Read the model definition and answer for the solid it produces. Units are mm, in the model's axes. Give positions to 0.01 mm unless a question says otherwise; leave off trailing zeros. Loops run counter-clockwise (first coordinate to the right, second up) from the corner with the lowest first, then second, coordinate; pieces in that order, holes last. Notation, with made-up numbers: (53.5, 30) - (88.5, 30) arc R19 ccw to (88.5, 34) - close; hole circle Ø4 at (55, -2). An arc over 180 degrees is marked (long way). Write item = value, one per line.
```python
from build123d import *

# Parameters (mm, degrees)
F0_W          = 158.75
F0_H          = 508
F1_DEPTH      = 158.75
F3_W          = 38.1
F3_H          = 114.3
F4_DEPTH      = 25.4
F2_W          = 31.75
F2_H          = 114.3
F5_DEPTH      = 25.4
F6_R          = 78.74
F7_SIZE       = 50.8
F8_W          = 38.1
F8_H          = 114.3
F9_DEPTH      = 25.4
F10_T2_ANGLE  = 90
F10_T4_ANGLE  = 90
F10_T6_ANGLE  = 90
F10_T8_ANGLE  = 90
F10_T12_DEPTH = 655.32
F10_T17_DEPTH = 655.32
F10_T23_DEPTH = 655.32
F10_T28_DEPTH = 655.32
F10_T33_DEPTH = 655.32
F10_T38_DEPTH = 655.32
F10_T43_DEPTH = 655.32
F10_T48_DEPTH = 655.32
F10_T53_DEPTH = 655.32
F10_T58_DEPTH = 655.32
F10_T63_DEPTH = 655.32
F10_T69_DEPTH = 655.32


# Not quite as in the source:
# - a fillet or chamfer that OpenCascade refuses, or shapes differently, is made with other operations: its cross-section is extruded or revolved along the edge and cut away or added


with BuildPart() as f1:
    # F0 (on Front) → F1 (new body)
    with BuildSketch(Plane.XZ):
        Rectangle(F0_W, F0_H)
    extrude(amount=F1_DEPTH)

    # F3 (on face) → F4 (join)
    with BuildSketch(Plane.YZ.offset(79.375)):
        with Locations((-79.375, 0)):
            Rectangle(F3_W, F3_H)
    extrude(amount=F4_DEPTH)

    # F2 (on face) → F5 (join)
    with BuildSketch(Plane.XZ.offset(158.75)):
        Rectangle(F2_W, F2_H)
    extrude(amount=F5_DEPTH)

    # F6
    f6_edges = [f1.edges().sort_by_distance(p)[0] for p in [
        (79.375, -79.375, 254),
        (-79.375, -79.375, 254),
        (0, 0, 254),
        (0, -158.75, 254),
    ]]
    fillet(f6_edges, radius=F6_R)

    # F7
    f7_edges = [f1.edges().sort_by_distance(p)[0] for p in [
        (-79.375, -79.375, -254),
        (79.375, -79.375, -254),
        (0, 0, -254),
        (0, -158.75, -254),
    ]]
    chamfer(f7_edges, length=F7_SIZE)

    # F8 (on face) → F9 (join)
    with BuildSketch(Plane(origin=(0, 0, 0), x_dir=(-1, 0, 0), z_dir=(0, 1, 0))):
        Rectangle(F8_W, F8_H)
    extrude(amount=F9_DEPTH)

    # F10: fillet of radius 79.248 on 4 edges, made by hand

    # F10_s1 → F10_t2 (revolve, cut)
    with BuildSketch(Plane.YZ.offset(0.127)):
        with BuildLine():
            ThreePointArc((-80.01, 254), (-135.6875879506, 230.9375879506), (-158.75, 175.26))
            Line((-158.75, 175.26), (-158.75, 254))
            Line((-158.75, 254), (-80.01, 254))
        make_face()
    revolve(axis=Axis((0.127, -79.502, 254), (0, 0, 1)), revolution_arc=F10_T2_ANGLE, mode=Mode.SUBTRACT)

    # F10_s3 → F10_t4 (revolve, cut)
    with BuildSketch(Plane.YZ.offset(-0.127)):
        with BuildLine():
            ThreePointArc((-78.74, 254), (-23.0624120494, 230.9375879506), (0, 175.26))
            Line((0, 175.26), (0, 254))
            Line((0, 254), (-78.74, 254))
        make_face()
    revolve(axis=Axis((-0.127, -79.248, 254), (0, 0, 1)), revolution_arc=F10_T4_ANGLE, mode=Mode.SUBTRACT)

    # F10_s5 → F10_t6 (revolve, cut)
    with BuildSketch(Plane.XZ.offset(79.502)):
        with BuildLine():
            ThreePointArc((-0.635, 254), (-56.3125879506, 230.9375879506), (-79.375, 175.26))
            Line((-79.375, 175.26), (-79.375, 254))
            Line((-79.375, 254), (-0.635, 254))
        make_face()
    revolve(axis=Axis((-0.127, -79.502, 254), (0, 0, 1)), revolution_arc=F10_T6_ANGLE, mode=Mode.SUBTRACT)

    # F10_s7 → F10_t8 (revolve, cut)
    with BuildSketch(Plane.XZ.offset(79.248)):
        with BuildLine():
            ThreePointArc((0.635, 254), (56.3125879506, 230.9375879506), (79.375, 175.26))
            Line((79.375, 175.26), (79.375, 254))
            Line((79.375, 254), (0.635, 254))
        make_face()
    revolve(axis=Axis((0.127, -79.248, 254), (0, 0, 1)), revolution_arc=F10_T8_ANGLE, mode=Mode.SUBTRACT)


with BuildPart() as f10_tool10:
    # F10_s11 → F10_t12 (new body)
    with BuildSketch(Plane.XY.offset(-401.32)):
        with BuildLine():
            ThreePointArc((0.127, 0), (56.1637981955, -23.2112018045), (79.375, -79.248))
            Line((79.375, -79.248), (79.375, 0))
            Line((79.375, 0), (0.127, 0))
        make_face()
    extrude(amount=F10_T12_DEPTH)

    split(bisect_by=Plane.XY.offset(-57.15), keep=Keep.BOTTOM)


with BuildPart() as f1_1:
    add(f1.part)

    # F10_t9: cut F10_tool10
    add(f10_tool10.part, mode=Mode.SUBTRACT)


with BuildPart() as f10_tool15:
    # F10_s16 → F10_t17 (new body)
    with BuildSketch(Plane.XY.offset(-401.32)):
        with BuildLine():
            ThreePointArc((0.127, 0), (56.1637981955, -23.2112018045), (79.375, -79.248))
            Line((79.375, -79.248), (79.375, 0))
            Line((79.375, 0), (0.127, 0))
        make_face()
    extrude(amount=F10_T17_DEPTH)

    split(bisect_by=Plane.YZ.offset(19.05), keep=Keep.TOP)

    split(bisect_by=Plane.XZ.offset(60.325), keep=Keep.BOTTOM)


with BuildPart() as f1_2:
    add(f1_1.part)

    # F10_t14: cut F10_tool15
    add(f10_tool15.part, mode=Mode.SUBTRACT)


with BuildPart() as f10_tool21:
    # F10_s22 → F10_t23 (new body)
    with BuildSketch(Plane.XY.offset(-401.32)):
        with BuildLine():
            ThreePointArc((0.127, 0), (56.1637981955, -23.2112018045), (79.375, -79.248))
            Line((79.375, -79.248), (79.375, 0))
            Line((79.375, 0), (0.127, 0))
        make_face()
    extrude(amount=F10_T23_DEPTH)

    split(bisect_by=Plane.XY.offset(57.15), keep=Keep.TOP)


with BuildPart() as f1_3:
    add(f1_2.part)

    # F10_t20: cut F10_tool21
    add(f10_tool21.part, mode=Mode.SUBTRACT)


with BuildPart() as f10_tool26:
    # F10_s27 → F10_t28 (new body)
    with BuildSketch(Plane.XY.offset(254)):
        with BuildLine():
            ThreePointArc((-79.375, -79.502), (-56.1637981955, -135.5387981955), (-0.127, -158.75))
            Line((-0.127, -158.75), (-79.375, -158.75))
            Line((-79.375, -158.75), (-79.375, -79.502))
        make_face()
    extrude(amount=-F10_T28_DEPTH)

    split(bisect_by=Plane.XY.offset(57.15), keep=Keep.TOP)


with BuildPart() as f1_4:
    add(f1_3.part)

    # F10_t25: cut F10_tool26
    add(f10_tool26.part, mode=Mode.SUBTRACT)


with BuildPart() as f10_tool31:
    # F10_s32 → F10_t33 (new body)
    with BuildSketch(Plane.XY.offset(254)):
        with BuildLine():
            ThreePointArc((-79.375, -79.502), (-56.1637981955, -135.5387981955), (-0.127, -158.75))
            Line((-0.127, -158.75), (-79.375, -158.75))
            Line((-79.375, -158.75), (-79.375, -79.502))
        make_face()
    extrude(amount=-F10_T33_DEPTH)

    split(bisect_by=Plane.YZ.offset(-15.875), keep=Keep.BOTTOM)


with BuildPart() as f1_5:
    add(f1_4.part)

    # F10_t30: cut F10_tool31
    add(f10_tool31.part, mode=Mode.SUBTRACT)


with BuildPart() as f10_tool36:
    # F10_s37 → F10_t38 (new body)
    with BuildSketch(Plane.XY.offset(254)):
        with BuildLine():
            ThreePointArc((-79.375, -79.502), (-56.1637981955, -135.5387981955), (-0.127, -158.75))
            Line((-0.127, -158.75), (-79.375, -158.75))
            Line((-79.375, -158.75), (-79.375, -79.502))
        make_face()
    extrude(amount=-F10_T38_DEPTH)

    split(bisect_by=Plane.XY.offset(-57.15), keep=Keep.BOTTOM)


with BuildPart() as f1_6:
    add(f1_5.part)

    # F10_t35: cut F10_tool36
    add(f10_tool36.part, mode=Mode.SUBTRACT)


with BuildPart() as f10_tool41:
    # F10_s42 → F10_t43 (new body)
    with BuildSketch(Plane.XY.offset(254)):
        with BuildLine():
            ThreePointArc((-79.375, -79.248), (-56.1637981955, -23.2112018045), (-0.127, 0))
            Line((-0.127, 0), (-79.375, 0))
            Line((-79.375, 0), (-79.375, -79.248))
        make_face()
    extrude(amount=-F10_T43_DEPTH)

    split(bisect_by=Plane.XY.offset(57.15), keep=Keep.TOP)


with BuildPart() as f1_7:
    add(f1_6.part)

    # F10_t40: cut F10_tool41
    add(f10_tool41.part, mode=Mode.SUBTRACT)


with BuildPart() as f10_tool46:
    # F10_s47 → F10_t48 (new body)
    with BuildSketch(Plane.XY.offset(254)):
        with BuildLine():
            ThreePointArc((-79.375, -79.248), (-56.1637981955, -23.2112018045), (-0.127, 0))
            Line((-0.127, 0), (-79.375, 0))
            Line((-79.375, 0), (-79.375, -79.248))
        make_face()
    extrude(amount=-F10_T48_DEPTH)

    split(bisect_by=Plane.YZ.offset(-19.05), keep=Keep.BOTTOM)


with BuildPart() as f1_8:
    add(f1_7.part)

    # F10_t45: cut F10_tool46
    add(f10_tool46.part, mode=Mode.SUBTRACT)


with BuildPart() as f10_tool51:
    # F10_s52 → F10_t53 (new body)
    with BuildSketch(Plane.XY.offset(254)):
        with BuildLine():
            ThreePointArc((-79.375, -79.248), (-56.1637981955, -23.2112018045), (-0.127, 0))
            Line((-0.127, 0), (-79.375, 0))
            Line((-79.375, 0), (-79.375, -79.248))
        make_face()
    extrude(amount=-F10_T53_DEPTH)

    split(bisect_by=Plane.XY.offset(-57.15), keep=Keep.BOTTOM)


with BuildPart() as f1_9:
    add(f1_8.part)

    # F10_t50: cut F10_tool51
    add(f10_tool51.part, mode=Mode.SUBTRACT)


with BuildPart() as f10_tool56:
    # F10_s57 → F10_t58 (new body)
    with BuildSketch(Plane.XY.offset(-401.32)):
        with BuildLine():
            ThreePointArc((0.127, -158.75), (56.1637981955, -135.5387981955), (79.375, -79.502))
            Line((79.375, -79.502), (79.375, -158.75))
            Line((79.375, -158.75), (0.127, -158.75))
        make_face()
    extrude(amount=F10_T58_DEPTH)

    split(bisect_by=Plane.XY.offset(-57.15), keep=Keep.BOTTOM)


with BuildPart() as f1_10:
    add(f1_9.part)

    # F10_t55: cut F10_tool56
    add(f10_tool56.part, mode=Mode.SUBTRACT)


with BuildPart() as f10_tool61:
    # F10_s62 → F10_t63 (new body)
    with BuildSketch(Plane.XY.offset(-401.32)):
        with BuildLine():
            ThreePointArc((0.127, -158.75), (56.1637981955, -135.5387981955), (79.375, -79.502))
            Line((79.375, -79.502), (79.375, -158.75))
            Line((79.375, -158.75), (0.127, -158.75))
        make_face()
    extrude(amount=F10_T63_DEPTH)

    split(bisect_by=Plane.YZ.offset(15.875), keep=Keep.TOP)

    split(bisect_by=Plane.XZ.offset(98.425), keep=Keep.TOP)


with BuildPart() as f1_11:
    add(f1_10.part)

    # F10_t60: cut F10_tool61
    add(f10_tool61.part, mode=Mode.SUBTRACT)


with BuildPart() as f10_tool67:
    # F10_s68 → F10_t69 (new body)
    with BuildSketch(Plane.XY.offset(-401.32)):
        with BuildLine():
            ThreePointArc((0.127, -158.75), (56.1637981955, -135.5387981955), (79.375, -79.502))
            Line((79.375, -79.502), (79.375, -158.75))
            Line((79.375, -158.75), (0.127, -158.75))
        make_face()
    extrude(amount=F10_T69_DEPTH)

    split(bisect_by=Plane.XY.offset(57.15), keep=Keep.TOP)


with BuildPart() as f1_12:
    add(f1_11.part)

    # F10_t66: cut F10_tool67
    add(f10_tool67.part, mode=Mode.SUBTRACT)


solid = f1_12.part
```
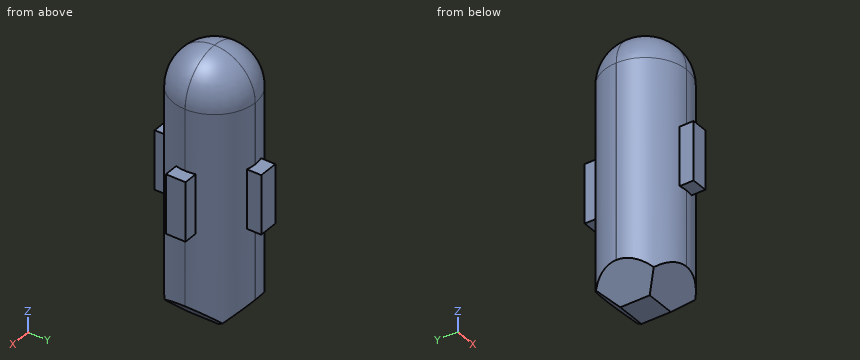
1) A cutting plane is placed at C-C on z = -141.5. Determine the outline of the cut face in (x, y) (3 decimals), then the cut area to 3 significant figures.
Output:
outline = (-79.375, -79.502) arc R79.248 ccw to (-0.127, -158.75) - (0.127, -158.75) arc R79.248 ccw to (79.375, -79.502) - (79.375, -79.248) arc R79.248 ccw to (0.127, 0) - (-0.127, 0) arc R79.248 ccw to (-79.375, -79.248) - close
area = 19,800 mm²
2) Find the intervals of material crossed by probe 1 along Y at (x, z) = (2.5, -127); probe 2 along Z at (x, y) = (-14.5, 10); probe 3 along Y at (x, z) = (-51.5, -103), in increasing order.
Output:
probe_1 = -158.71 to -0.04
probe_2 = -57.15 to 57.15
probe_3 = -139.84 to -18.91
3) A cutting plane is placed at A-A on z = -23. Determine the outline of the cut face in (x, y) (3 decimals).
Output:
outline = (-79.375, -79.502) arc R79.248 ccw to (-15.875, -157.17) - (-15.875, -184.15) - (15.875, -184.15) - (15.875, -157.17) arc R79.248 ccw to (77.083, -98.425) - (104.775, -98.425) - (104.775, -60.325) - (77.083, -60.325) arc R79.248 ccw to (19.05, -2.292) - (19.05, 25.4) - (-19.05, 25.4) - (-19.05, -2.292) arc R79.248 ccw to (-79.375, -79.248) - close
4) Each of these flat-tipped pins is pushed along its axis until it touches: P1, Ø1.5, axis at x = 69.5, z = -192.5, coming from the +Y side; P2, Ø21.5, axis at y = -177, z = 9, coming from the -X side (3 decimals); P3, Ø22, axis at y = 14, z = -3, coming from the -X side. Where does it stop, or does it pass through?
Output:
P1 = -39.61
P2 = -15.875
P3 = -19.05
5) A cutting plane is placed at B-B on x = 93. Determine the outline of the cut face in (y, z) (3 decimals), then the cut area to 3 significant figures.
Output:
outline = (-98.425, -57.15) - (-60.325, -57.15) - (-60.325, 57.15) - (-98.425, 57.15) - close
area = 4,350 mm²
